Can you work these out from the drawing? Everything is in mm from the part's minimum corner. Coordinates: 2 decimals unless noted, no trailing zeros. Order: outer loops, then holes, each group sorted by start corner. A loop starts at its lowest first (then second) coordinate and runs counter-clockwise, first axis right, second up. Notation, with made-up numbers: (-32, 88) - (25, 88) arc R22 cw to (25, 124) - close; hole circle Ø6 at (33.5, -29). An arc over 180 degrees is marked (long way). One line per item, written item: value.
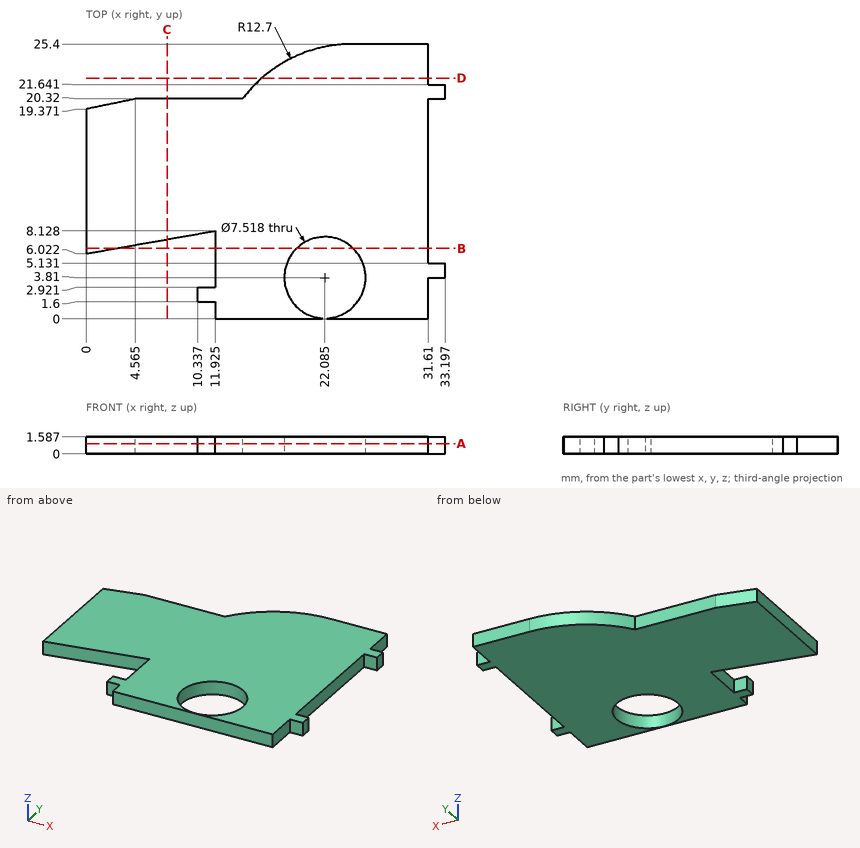
Item 1: If I drill on probe 1 along Y at (x, z) = (32, 1.2); probe 2 along X at (y, z) = (9.75, 0.9); probe 3 along X at (y, z) = (5.25, 1.3) (1 decimal), over which ranges is the centre line in solid material (lowest first)?
Conclusion:
probe 1: 3.81 to 5.13, 20.32 to 21.64
probe 2: 0 to 31.61
probe 3: 11.9 to 18.6, 25.6 to 31.6
Item 2: I'm going to push flat-ended pins straight in: pin 1 Ø0.5 at (y, z) = (1, 1) entering from -X (1 decimal); pin 2 Ø0.8 at (y, z) = (11, 1) entering from +X; pin 3 Ø0.8 at (x, z) = (11, 1) entering from -Y. Where does each tip first touch, or does it pass through?
Conclusion:
pin 1: x = 11.9
pin 2: x = 31.61
pin 3: y = 1.6
Item 3: I want a section at B-B on y = 6.5. Please give me the cut outline in (x, z) (1 decimal).
Conclusion:
outline: (0, 0) - (2.7, 0) - (2.7, 1.6) - (0, 1.6) - close; (11.9, 0) - (19.5, 0) - (19.5, 1.6) - (11.9, 1.6) - close; (24.7, 0) - (31.6, 0) - (31.6, 1.6) - (24.7, 1.6) - close
Item 4: I want a section at C-C on x = 7.5. Please give me the cut outline in (y, z).
Conclusion:
outline: (7.35, 0) - (20.32, 0) - (20.32, 1.59) - (7.35, 1.59) - close
Item 5: I want a section at A-A on z = 0.95. Please give me the cut outline in (x, y) (1 decimal).
Conclusion:
outline: (0, 6) - (11.9, 8.1) - (11.9, 2.9) - (10.3, 2.9) - (10.3, 1.6) - (11.9, 1.6) - (11.9, 0) - (31.6, 0) - (31.6, 3.8) - (33.2, 3.8) - (33.2, 5.1) - (31.6, 5.1) - (31.6, 20.3) - (33.2, 20.3) - (33.2, 21.6) - (31.6, 21.6) - (31.6, 25.4) - (24.6, 25.4) arc R12.7 ccw to (14.5, 20.3) - (4.6, 20.3) - (0, 19.4) - close; hole circle Ø7.5 at (22.1, 3.8)
Item 6: I want a section at D-D on y = 22.25. Please give me the cut outline in (x, z).
Conclusion:
outline: (16.25, 0) - (31.61, 0) - (31.61, 1.59) - (16.25, 1.59) - close
